Source: CAD feature listing. Evaluate the final solid. Frame: model axes, mm. Round coordinates to 2 decimals unless told otherwise and drop trailing zeros. Write item = value, one per line. Start each with the question number.
(1) Contact query for flat-ended pins moving along their axis: pin 1 Ø5 at (x, y) = (0, 0) entering from +Z; pin 2 Ø6 at (x, z) = (-25, 5.5) entering from +Y; pin 3 Ø1 at (x, z) = (-35, 28.5) entering from -Y; pin 4 Ø12 at (x, z) = (38, 21) entering from -Y. Output: stop coordinate, or through.
(2) Cut plane A-A on y = 0. Give the number of separate pieces and of enclosed holes in the cut face, then the cut area to 3 significant figures.
(3) Ray query, line 1 (Y direction, x = 0, z = 16); line 2 (Y direction, x = 3, z = 32); line 3 (Y direction, x = -44.5, z = 31.5). Return the intervals inside material, ascending.
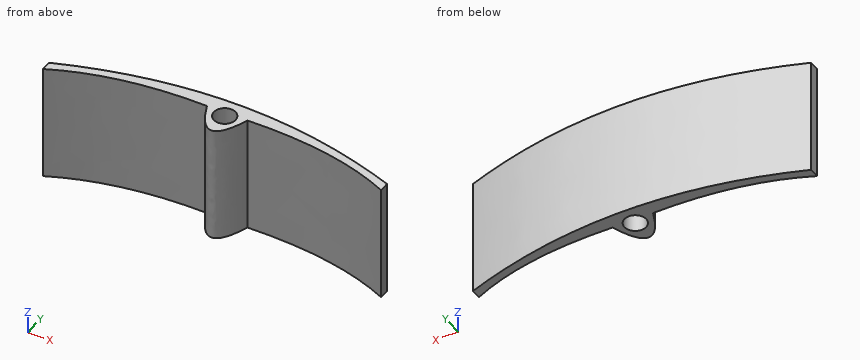
from build123d import *

# Parameters (mm, degrees)
SKETCH_1_R      = 3.25
EXTRUDE_1_DEPTH = 35


with BuildPart() as part:
    # 草圖1 → 填料-伸長1 (new body)
    with BuildSketch(Plane.XY):
        with BuildLine():
            Line((-50, -3.480646824), (-50, -6.480646824))
            add(Edge.make_bspline(
                [(-6, 1.314323068), (-31.607950909, 1.920554197), (-50, -6.480646824)],
                knots=[0, 0, 0, 1, 1, 1], degree=2))
            add(Edge.make_bspline(
                [(-6, 1.314323068), (0, -15), (6, 1.314323068)],
                knots=[0, 0, 0, 1, 1, 1], degree=2))
            add(Edge.make_bspline(
                [(6, 1.314323068), (32.228671013, 1.920554197), (50, -6.480646824)],
                knots=[0, 0, 0, 1, 1, 1], degree=2))
            Line((50, -6.480646824), (50, -3.480646824))
            add(Edge.make_bspline(
                [(-50, -3.480646824), (0, 15), (50, -3.480646824)],
                knots=[0, 0, 0, 1, 1, 1], degree=2))
        make_face()
        Circle(SKETCH_1_R, mode=Mode.SUBTRACT)
    extrude(amount=EXTRUDE_1_DEPTH)


solid = part.part
Evaluation:
q1.pin_1 = through
q1.pin_2 = 3.97
q1.pin_3 = -1.52
q1.pin_4 = -3.99
q2.separate_pieces = 4
q2.enclosed_holes = 0
q2.area = 962 mm^2
q3.line_1 = -6.84 to -3.25, 3.25 to 5.76
q3.line_2 = -4.8 to -1.25, 1.25 to 5.73
q3.line_3 = -4.23 to -1.56
